Can you work these out from the model? Positions are in its coordinate system, mm. Face numbers are marked on the shaded views. Give positions to 0.01 mm unless a question says otherwise; leave off trailing zeros. Order: outer loops, then holes, each group sorted by start corner. A loop starts at its lowest first (then second) coordinate and runs counter-clockwise, first axis right, second up. Notation, with made-up numbers: M 22.5,-20 L 29.5,-20 A19 cw 29.5,-11 Z; hole C -34.5,-17.75 d9. An arc over 180 degrees is marked long. Write each question's results on one line, items separated by ' | '.
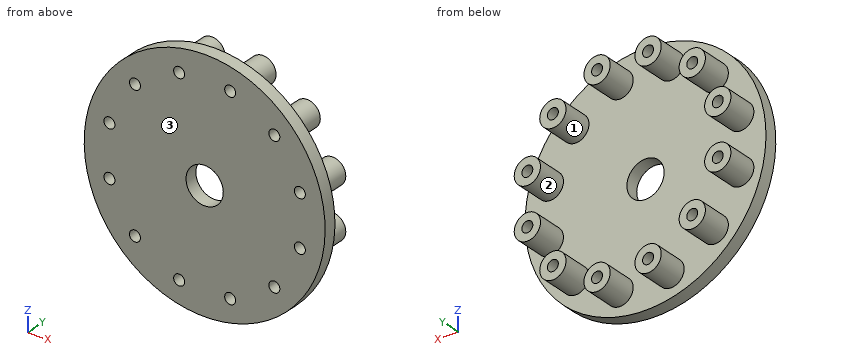
from build123d import *

# Parameters (mm, degrees)
SKETCH1_R           = 27.5
SKETCH1_R_2         = 3
SKETCH1_R_3         = 4.25
BOSS_EXTRUDE1_DEPTH = 3
SKETCH2_R           = 3
BOSS_EXTRUDE2_DEPTH = 10
M3_TAPPED_HOLE1_D   = 2.5
CIRPATTERN1_COUNT   = 12


with BuildPart() as part:
    # Sketch1 → Boss-Extrude1 (new body)
    with BuildSketch(Plane(origin=(0, 0, 0), x_dir=(1, 0, 0), z_dir=(0, 1, 0))):
        with Locations(Location((0, 0, 0), (0, 0, 270))):
            Circle(SKETCH1_R)
        with Locations(Location((21.733331092, -5.823428515, 0), (0, 0, 270))):
            Circle(SKETCH1_R_2, mode=Mode.SUBTRACT)
        with Locations(Location((15.909902577, -15.909902577, 0), (0, 0, 270))):
            Circle(SKETCH1_R_2, mode=Mode.SUBTRACT)
        with Locations(Location((5.823428515, -21.733331092, 0), (0, 0, 270))):
            Circle(SKETCH1_R_2, mode=Mode.SUBTRACT)
        with Locations(Location((-5.823428515, -21.733331092, 0), (0, 0, 270))):
            Circle(SKETCH1_R_2, mode=Mode.SUBTRACT)
        with Locations(Location((-15.909902577, -15.909902577, 0), (0, 0, 270))):
            Circle(SKETCH1_R_2, mode=Mode.SUBTRACT)
        with Locations(Location((-21.733331092, -5.823428515, 0), (0, 0, 270))):
            Circle(SKETCH1_R_2, mode=Mode.SUBTRACT)
        with Locations(Location((-21.733331092, 5.823428515, 0), (0, 0, 270))):
            Circle(SKETCH1_R_2, mode=Mode.SUBTRACT)
        with Locations(Location((-15.909902577, 15.909902577, 0), (0, 0, 270))):
            Circle(SKETCH1_R_2, mode=Mode.SUBTRACT)
        with Locations(Location((-5.823428515, 21.733331092, 0), (0, 0, 270))):
            Circle(SKETCH1_R_2, mode=Mode.SUBTRACT)
        with Locations(Location((5.823428515, 21.733331092, 0), (0, 0, 270))):
            Circle(SKETCH1_R_2, mode=Mode.SUBTRACT)
        with Locations(Location((15.909902577, 15.909902577, 0), (0, 0, 270))):
            Circle(SKETCH1_R_2, mode=Mode.SUBTRACT)
        with Locations(Location((21.733331092, 5.823428515, 0), (0, 0, 270))):
            Circle(SKETCH1_R_2, mode=Mode.SUBTRACT)
        with Locations(Location((0, 0, 0), (0, 0, 270))):
            Circle(SKETCH1_R_3, mode=Mode.SUBTRACT)
    extrude(amount=BOSS_EXTRUDE1_DEPTH)

    # Sketch2 → Boss-Extrude2 (add)
    with BuildSketch(Plane.XZ):
        with Locations(Location((15.909902577, 15.909902577, 0), (0, 0, 270))):
            Circle(SKETCH2_R)
        with Locations(Location((21.733331092, 5.823428515, 0), (0, 0, 270))):
            Circle(SKETCH2_R)
        with Locations(Location((21.733331092, -5.823428515, 0), (0, 0, 270))):
            Circle(SKETCH2_R)
        with Locations(Location((15.909902577, -15.909902577, 0), (0, 0, 270))):
            Circle(SKETCH2_R)
        with Locations(Location((5.823428515, -21.733331092, 0), (0, 0, 270))):
            Circle(SKETCH2_R)
        with Locations(Location((-5.823428515, -21.733331092, 0), (0, 0, 270))):
            Circle(SKETCH2_R)
        with Locations(Location((-15.909902577, -15.909902577, 0), (0, 0, 270))):
            Circle(SKETCH2_R)
        with Locations(Location((-21.733331092, -5.823428515, 0), (0, 0, 270))):
            Circle(SKETCH2_R)
        with Locations(Location((-21.733331092, 5.823428515, 0), (0, 0, 270))):
            Circle(SKETCH2_R)
        with Locations(Location((-15.909902577, 15.909902577, 0), (0, 0, 270))):
            Circle(SKETCH2_R)
        with Locations(Location((-5.823428515, 21.733331092, 0), (0, 0, 270))):
            Circle(SKETCH2_R)
        with Locations(Location((5.823428515, 21.733331092, 0), (0, 0, 270))):
            Circle(SKETCH2_R)
    extrude(amount=-BOSS_EXTRUDE2_DEPTH)

    # M3 Tapped Hole1 (through all)
    with Locations(Plane(origin=(0, 10, 0), x_dir=(1, 0, 0), z_dir=(0, 1, 0))):
        with Locations((-5.823428515, 21.733331092)):
            m3_tapped_hole1 = Hole(M3_TAPPED_HOLE1_D / 2)

    # CirPattern1: M3 Tapped Hole1 ×12 about axis
    cirpattern1_axis = Axis((0, 0, 0), (0, 1, 0))
    for i in range(1, CIRPATTERN1_COUNT):
        add(m3_tapped_hole1.rotate(cirpattern1_axis, i * 360 / CIRPATTERN1_COUNT), mode=Mode.SUBTRACT)


solid = part.part
(1) Imagine slicing it at A-A, the plane z = 0. Write out the boundary of the cut face in (x, y).
Data:
outline: M -27.5,0 L -4.25,0 L -4.25,3 L -27.5,3 Z; M 4.25,0 L 27.5,0 L 27.5,3 L 4.25,3 Z
(2) Imagine slicing it at B-B, the plane y = 9. Count the separate pieces of the cut face and the enclosed holes in it, plus the area to 3 significant figures.
Data:
separate pieces: 12 | enclosed holes: 12 | area: 280 mm2
(3) Imagine slicing it at D-D, the plane z = 5.5. Write out the boundary of the cut face in (x, y).
Data:
outline: M -26.94,0 L -22.94,0 L -22.94,10 L -24.72,10 L -24.72,3 L -26.94,3 Z; M -20.53,0 L 20.53,0 L 20.53,10 L 18.75,10 L 18.75,3 L -18.75,3 L -18.75,10 L -20.53,10 Z; M 22.94,0 L 26.94,0 L 26.94,3 L 24.72,3 L 24.72,10 L 22.94,10 Z
(4) We'd pull the mould along Z, two halves only. Please class the marked faces 1, 2 and 3: +Z half, -Z half, draft (parallel to the pull), parting line (faces both ways), or undercut.
Data:
face 1: undercut | face 2: undercut | face 3: draft
(5) I need wall thicknesses on L1, parallel to X at y = 4.5, z = 16; L2, parallel to Z at x = 19, y = 8; L3, parallel to X at y = 4.25, z = 21. Which ranges of each line are inside material? Lowest first, please. Write a range as from..to.
Data:
L1: x = -18.91..-17.16, -14.66..-12.91, 12.91..14.66, 17.16..18.91 | L2: z = -7.06..-4.59, 4.59..7.06 | L3: x = -8.73..-6.84, -4.81..-2.91, 2.91..4.81, 6.84..8.73
(6) Will these pins go through, and if not, where does the flat tip stop? P1, Ø3, axis at x = 5.82, z = 21.73, coming from the +Y side; P2, Ø1.5, axis at x = -21.73, z = 5.82, coming from the +Y side; P3, Ø1.5, axis at x = -4.5, z = -11.5, coming from the +Y side; P4, Ø6, axis at y = 3, z = -16, coming from the +X side.
Data:
P1: stops at y = 10 | P2: passes through | P3: stops at y = 3 | P4: stops at x = 24.23
(7) Imagine slicing it at C-C, the plane x = 0. Write out the boundary of the cut face in (y, z), plus the area to 4 significant figures.
Data:
outline: M 0,-27.5 L 3,-27.5 L 3,-4.25 L 0,-4.25 Z; M 0,4.25 L 3,4.25 L 3,27.5 L 0,27.5 Z | area: 139.5 mm2
